For this review, take the finished solid that the model builds, in its own axes (mm). Face numbers are marked on the shaded views. Give positions to 0.01 mm unless a question says otherwise; leave off trailing zeros. Write each loop counter-clockwise with the first axis right and the second up, starting at its lowest first coordinate (ties: lowest second). Pieces come first, ordered by that corner, then holes. Notation, with made-up numbers: M 66.5,4.5 L 116.5,4.5 A13 cw 116.5,23.5 Z; hole C 34,18 d3. An arc over 180 degrees is marked long. Use one line per item in the form item = value. Start each with the question number.
Q1. Consider section B-B on z = 0. Write out the cut boundary in (x, y), and give its area (3 significant figures).
Q2. Clearance check with flat-ended pins moving along their axes: pin 1 Ø1.5 at (x, z) = (-6, -3.5) entering from -Y; pin 2 Ø1.5 at (y, z) = (2.5, -7.5) entering from -X; pin 3 Ø5.5 at (x, z) = (0, 0) entering from -Y. State where each tip first meets the part, or that it passes through.
Q3. For probe 1 along Z at (x, y) = (0, 2.95); probe 2 along Z at (x, y) = (-0.75, 1.5); probe 3 along X at (y, z) = (1.5, 1.75), list the stretches that pass through material, from the lowest coordinate up. Write a range as [from, to].
Q4. Consider section D-D on z = -5.25. Write out the cut boundary in (x, y), and give its area (3 significant figures).
Q5. Mouldability with a two-part tool opening along Z and no side actions: class the marked faces 1, 2 and 3 as released by +Z, released by -Z, zero draft, split by the parting line, or undercut.
Q6. Consider section A-A on x = 0. Write out the cut boundary in (y, z).
Q7. Consider section C-C on y = 5.25. Write out the cut boundary in (x, z), and give its area (3 significant figures).
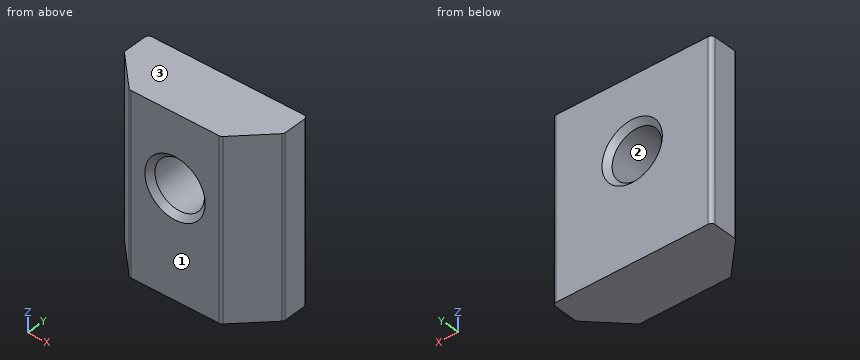
Autodesk Inventor part; units mm, degrees
ref_plane "tnut_XY" through (0, 6.1595, 0) normal (0, 1, 0) x (1, 0, 0)
ref_plane "tnut_YZ" through (0, 6.1595, 0) normal (1, 0, 0) x (0, 0, -1)
ref_plane "tnut_ZX" through (0, 6.1595, 0) normal (0, 0, -1) x (0, 1, 0)
sketch "Sketch_1" plane through (0, 0, -10.6426) normal (0, 0, 1) x (1, 0, 0)
  line L0 (-7.9375, 5.7785) -> (-7.9375, 3.5455)
  arc A0 (-7.9375, 3.5455) -> (-7.8259, 3.2761) centre (-7.5565, 3.5455) ccw
  line L1 (-7.8259, 3.2761) -> (-4.6614, 0.1116)
  arc A1 (-4.6614, 0.1116) -> (-4.392, 0) centre (-4.392, 0.381) ccw
  line L2 (-4.392, 0) -> (4.392, 0)
  arc A2 (4.392, 0) -> (4.6614, 0.1116) centre (4.392, 0.381) ccw
  line L3 (4.6614, 0.1116) -> (7.8259, 3.2761)
  arc A3 (7.8259, 3.2761) -> (7.9375, 3.5455) centre (7.5565, 3.5455) ccw
  line L4 (7.9375, 3.5455) -> (7.9375, 5.7785)
  arc A4 (7.9375, 5.7785) -> (7.5565, 6.1595) centre (7.5565, 5.7785) ccw
  line L5 (7.5565, 6.1595) -> (-7.5565, 6.1595)
  arc A5 (-7.5565, 6.1595) -> (-7.9375, 5.7785) centre (-7.5565, 5.7785) ccw
extrude "Extrusion1" add sketch "Sketch_1" along normal blind 17.78
sketch "Sketch_4" plane through (0, 0, 0) normal (0, 0, 1) x (1, 0, 0)
  line L0 (0, 0) -> (0, 6.1595)
  line L1 (0, 6.1595) -> (3, 6.1595)
  line L2 (3, 6.1595) -> (2.4585, 5.618)
  line L3 (2.4585, 5.618) -> (2.4585, 0.5415)
  line L4 (2.4585, 0.5415) -> (3, 0)
  line L5 (3, 0) -> (0, 0)
  line L6 (0, 0) -> (0, 6.1595)
revolve "Revolution1" cut sketch "Sketch_4" angle 360 about axis through (0, 0, 0) along (0, -1, 0)
thread "Thread1"
ref_plane "tnut_XY" through (0, 6.1595, 0) normal (0, 1, 0) x (1, 0, 0)
ref_plane "tnut_YZ" through (0, 6.1595, 0) normal (1, 0, 0) x (0, 0, -1)
ref_plane "tnut_ZX" through (0, 6.1595, 0) normal (0, 0, -1) x (0, 1, 0)
properties part number "40-1964"
Working result:
q1.outline = M -7.94,3.55 A0.38 ccw -7.83,3.28 L -4.66,0.11 A0.38 ccw -4.39,0 L -3,0 L -2.46,0.54 L -2.46,5.62 L -3,6.16 L -7.56,6.16 A0.38 ccw -7.94,5.78 Z; M 2.46,0.54 L 3,0 L 4.39,0 A0.38 ccw 4.66,0.11 L 7.83,3.28 A0.38 ccw 7.94,3.55 L 7.94,5.78 A0.38 ccw 7.56,6.16 L 3,6.16 L 2.46,5.62 Z
q1.area = 55.4 mm²
q2.pin_1 = 0.7
q2.pin_2 = -7.8
q2.pin_3 = 0.25
q3.probe_1 = [-10.64, -2.46], [2.46, 7.14]
q3.probe_2 = [-10.64, -2.34], [2.34, 7.14]
q3.probe_3 = [-6.05, -1.73], [1.73, 6.05]
q4.outline = M -7.94,3.55 A0.38 ccw -7.83,3.28 L -4.66,0.11 A0.38 ccw -4.39,0 L 4.39,0 A0.38 ccw 4.66,0.11 L 7.83,3.28 A0.38 ccw 7.94,3.55 L 7.94,5.78 A0.38 ccw 7.56,6.16 L -7.56,6.16 A0.38 ccw -7.94,5.78 Z
q4.area = 86.2 mm²
q5.face_1 = zero draft
q5.face_2 = undercut
q5.face_3 = released by +Z
q6.outline = M 0,-10.64 L 6.16,-10.64 L 6.16,-3 L 5.62,-2.46 L 0.54,-2.46 L 0,-3 Z; M 0,3 L 0.54,2.46 L 5.62,2.46 L 6.16,3 L 6.16,7.14 L 0,7.14 Z
q7.outline = M -7.94,-10.64 L 7.94,-10.64 L 7.94,7.14 L -7.94,7.14 Z; hole C 0,0 d4.92
q7.area = 263 mm²
